Answer from the drawing. Dimensions are ordinates in mm from the lowest x, y and z of the part. A direction names the side the tool comes from. Coordinates: 2 decimals unless noted, no trailing zeros. Order: outer loops, then holes, each group sorted by start corner. A loop starts at its lowest first (then second) coordinate and runs counter-clockwise, first axis right, second up. Notation, with made-up numbers: M -29,-37.75 L -4,-37.75 A14 ccw -4,-30.75 Z; hole C 25,-18.5 d3. An arc over 180 degrees is marked long. One line per question, with ' | ' between items. Start each with the question number.
1) Given P1, Ø2.5, axis at x = 10, z = 3.5, coming from the -Y side, flat-ended and moving along its own axis, determine where the tip first touches the part or whether it passes through.
2) Find section A-A, the plane x = 63. Write down the section's boundary in (y, z).
3) Find section D-D, the plane y = 10.5. Write down the section's boundary in (x, z).
4) Find section C-C, the plane z = 0.65. Count the separate pieces of the cut face and the enclosed holes in it, plus the area to 3 significant figures.
5) The mould has two halves that part along Y. Classify the marked faces 6, 7, 8 and 9: +Y half, -Y half, draft (parallel to the pull), parting line (faces both ways), or undercut.
6) Find section B-B, the plane y = 2.75. Write down the section's boundary in (x, z), plus the area to 3 significant figures.
7) A tool of negligible diameter and unlimited length cuts with its end or side. For the marked faces 1, 2, 3, 4 and 5, from which of +Z, -Z, +X, -X, +Y, -Y can it reach the whole face along a straight path? Write none if from no direction.
8) Consider probe 1 along X at (y, z) = (4, 4.05); probe 2 along X at (y, z) = (15, 3.7) (1 decimal); probe 3 along Y at (x, z) = (63, 3.6). Determine where each line is inside the solid, lowest interval first.
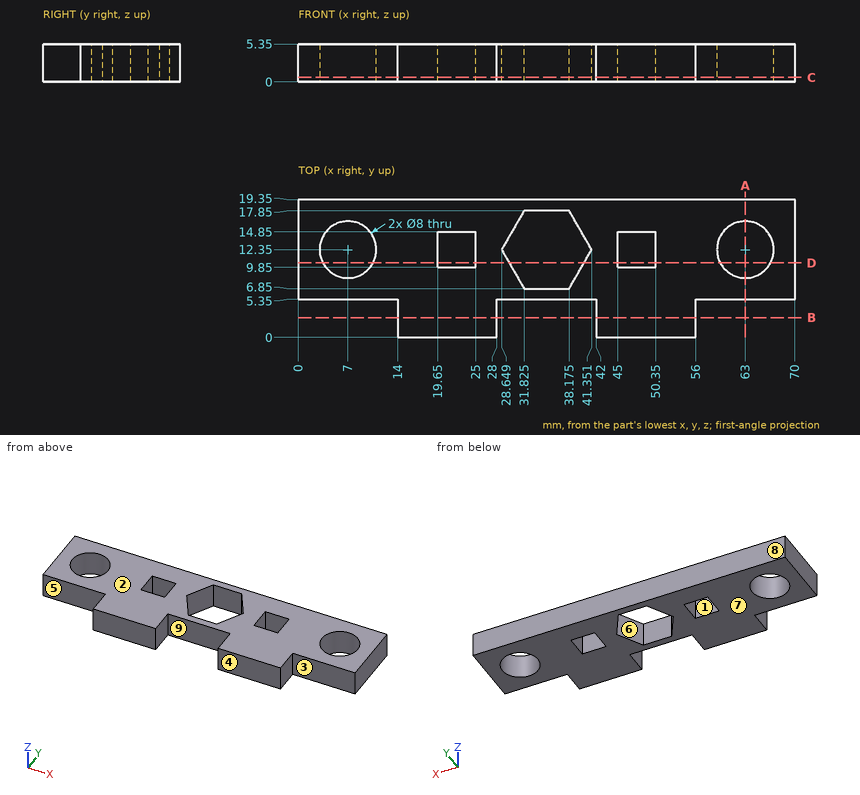
Report:
1) P1: stops at y = 5.35
2) outline: M 5.35,0 L 8.35,0 L 8.35,5.35 L 5.35,5.35 Z; M 16.35,0 L 19.35,0 L 19.35,5.35 L 16.35,5.35 Z
3) outline: M 0,0 L 3.45,0 L 3.45,5.35 L 0,5.35 Z; M 10.55,0 L 19.65,0 L 19.65,5.35 L 10.55,5.35 Z; M 25,0 L 29.72,0 L 29.72,5.35 L 25,5.35 Z; M 40.28,0 L 45,0 L 45,5.35 L 40.28,5.35 Z; M 50.35,0 L 59.45,0 L 59.45,5.35 L 50.35,5.35 Z; M 66.55,0 L 70,0 L 70,5.35 L 66.55,5.35 Z
4) separate pieces: 1 | enclosed holes: 5 | area: 871 mm^2
5) face 6: undercut | face 7: draft | face 8: +Y half | face 9: -Y half
6) outline: M 14,0 L 28,0 L 28,5.35 L 14,5.35 Z; M 42,0 L 56,0 L 56,5.35 L 42,5.35 Z | area: 150 mm^2
7) face 1: +Z, -Z | face 2: +Z, +X, -X, +Y, -Y | face 3: +Z, -Z, +X, -Y | face 4: +Z, -Z, +X, -X, -Y | face 5: +Z, -Z, -X, -Y
8) probe 1: x = 14 to 28, 42 to 56 | probe 2: x = 0 to 4, 10 to 30.2, 39.8 to 60, 66 to 70 | probe 3: y = 5.35 to 8.35, 16.35 to 19.35
